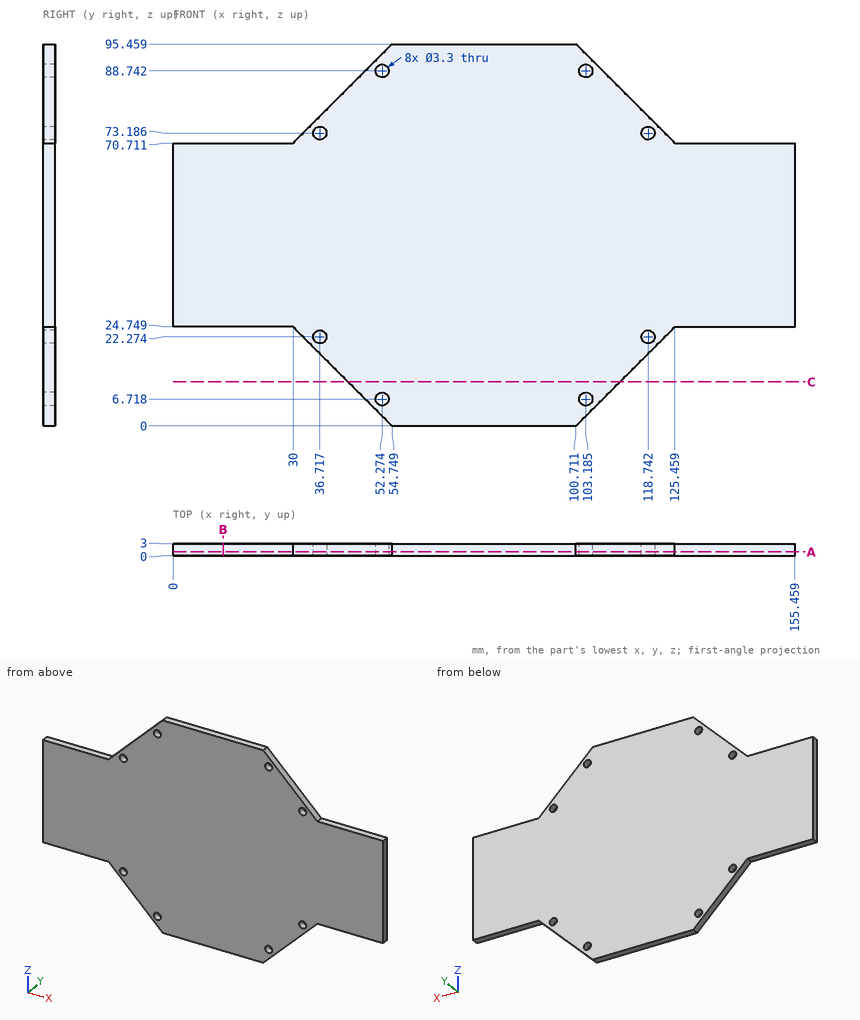
Here's the drawing with two shaded views (mm, measured from the low corner). I have some questions. Round coordinates to 2 decimals unless told otherwise and drop trailing zeros. Write each loop counter-clockwise with the first axis right and the second up, starting at its lowest first coordinate (ties: lowest second). Pieces come first, ordered by that corner, then holes. Notation, with made-up numbers: M 11.5,68.5 L 32.5,68.5 A20 cw 32.5,85.5 Z; hole C 51.5,72.25 d11. An arc over 180 degrees is marked long. Answer in a Markdown table with one row per item. Add a question column.
Q1. Imagine slicing it at A-A (y = 1). Give the number of separate pieces and of enclosed holes in the cut face, then the cut area to 3 significant figures.
Q2. Will these pins go through, and if not, where does the flat tip stop? pin 1 Ø0.9 at (x, y) = (11, 2) entering from -Z; pin 2 Ø8 at (x, z) = (24.5, 44.5) entering from -Y; pin 3 Ø2.5 at (x, z) = (36.72, 73.19) entering from +Y; pin 4 Ø1.5 at (x, y) = (21.5, 2) entering from +Z.
Q3. Imagine slicing it at C-C (z = 11). Please give me the cut outline in (x, y), then the cut area to 3 significant figures.
Q4. Imagine slicing it at B-B (x = 12.5). Please give me the cut outline in (y, z), then the cut area to 3 significant figures.
Q5. If I drill on line 1 (Z direction, x = 37, y = 0.5); line 2 (X direction, y = 1.8, z = 72) (1 decimal); line 3 (Z direction, x = 141.5, y = 0.85), over which ranges is the centre line in solid material (lowest first)? Write a range as from..to.
Values:
| question | item | result |
|---|---|---|
| 1 | separate pieces | 1 |
| 1 | enclosed holes | 8 |
| 1 | area | 10,600 mm^2 |
| 2 | pin 1 | z = 24.75 |
| 2 | pin 2 | y = 0 |
| 2 | pin 3 | through |
| 2 | pin 4 | z = 70.71 |
| 3 | outline | M 43.75,0 L 111.71,0 L 111.71,3 L 43.75,3 Z |
| 3 | area | 204 mm^2 |
| 4 | outline | M 0,24.75 L 3,24.75 L 3,70.71 L 0,70.71 Z |
| 4 | area | 138 mm^2 |
| 5 | line 1 | 17.75..20.65, 23.9..71.56, 74.81..77.71 |
| 5 | line 2 | 31.3..35.6, 37.9..117.6, 119.9..124.2 |
| 5 | line 3 | 24.75..70.71 |
